Can you work these out from the model? Positions are in its coordinate system, mm. A direction names the side the tool comes from. Coordinates: 2 decimals unless noted, no trailing zeros. Order: outer loops, then holes, each group sorted by start corner. A loop starts at its lowest first (then second) coordinate and runs counter-clockwise, first axis right, second up. Notation, with made-up numbers: (42.25, 7.25) - (98.25, 7.25) arc R24 cw to (98.25, 34.25) - close; hole circle Ø8 at (15, 18.5). An arc over 180 degrees is marked (long way). Return JSON: item names as keys, results as strings. Group by question number.
1) Imagine slicing it at A-A (x = -30.48). Write out the boundary of the cut face in (y, z), and give its area (3 significant figures).
2) If I drill on line 1 along Z through (x, y) = (-30.5, 2); line 2 along Z through (x, y) = (-55, 20); line 3 along X through (y, z) = (12.5, 24), over which ranges is the centre line in solid material (lowest first)?
3) Imagine slicing it at D-D (y = 24). Write out the boundary of the cut face in (x, z), and give its area (3 significant figures).
4) Which directions (+Z, -Z, +X, -X, +Y, -Y) give clear straight access to the entire face, cutting with the end or side of a thin tool? Please do faces 1 (the face through (-38.1, 3, -12)), 2 (the face through (-41, 12.7, 13)), 3 (the face through (-60.07, 21.38, 13.27)).
5) For pin 1 Ø4 at (x, z) = (-30.5, -22) entering from -Y; pin 2 Ø1 at (y, z) = (9, -31) entering from +X; pin 3 Ø12.5 at (x, y) = (-56.5, 11.5) entering from +Z; pin 4 Ø6.5 at (x, z) = (-30.48, 25.4) entering from +Y, each with a flat end and sliding along its axis, tell me the tip position at first contact or that it passes through.
6) Imagine slicing it at B-B (y = 14.5). Write out the boundary of the cut face in (x, z), and give its area (3 significant figures).
7) Imagine slicing it at C-C (x = -49.5). Write out the boundary of the cut face in (y, z), and give its area (3 significant figures).
8) If we mould it in two halves opening along Z, with no side actions, what happens to faces 4 (the face through (-38.1, 3, 38)), 5 (the face through (-19, 3, 50.8)), 6 (the face through (-8.992, 1.805, -27.552))? For each: pulls with the +Z half, pulls with the -Z half, needs draft (parallel to the pull), parting line crosses it, or undercut.
```python
from build123d import *

# Parameters (mm, degrees)
EXTRUDE_THIN1_DEPTH                             = 50.8
CUT_EXTRUDE2_START                              = -7.35
SKETCH3_W                                       = 25.4
SKETCH3_H                                       = 25.4
CUT_EXTRUDE2_DEPTH                              = 27.4
LPATTERN1_COUNT                                 = 2
LPATTERN1_PITCH                                 = 50
CSK_FOR_10_FLAT_HEAD_MACHINE_SCREW1_D           = 5.1054
CSK_FOR_10_FLAT_HEAD_MACHINE_SCREW1_CSINK_D     = 9.779
CSK_FOR_10_FLAT_HEAD_MACHINE_SCREW1_CSINK_ANGLE = 82
LPATTERN2_COUNT                                 = 2
LPATTERN2_PITCH                                 = 50.8
LPATTERN2_COUNT_DIR2                            = 2
LPATTERN2_PITCH_DIR2                            = 22.86


with BuildPart() as part:
    # Sketch1 → Extrude-Thin1 (new body, symmetric)
    with BuildSketch(Plane.XY):
        with BuildLine():
            Line((0, 0), (-50.8, 0))
            ThreePointArc((-50.8, 0), (-59.780256121, 21.680256121), (-38.1, 12.7))
            Line((-38.1, 12.7), (-44.45, 12.7))
            ThreePointArc((-44.45, 12.7), (-55.290128061, 17.190128061), (-50.8, 6.35))
            Line((-50.8, 6.35), (0, 6.35))
            Line((0, 6.35), (0, 0))
        make_face()
    extrude(amount=EXTRUDE_THIN1_DEPTH, both=True)

    # Sketch3 → Cut-Extrude2 (cut)
    with BuildSketch(Plane(origin=(0, 6.35, 0), x_dir=(1, 0, 0), z_dir=(0, 1, 0)).offset(CUT_EXTRUDE2_START)):
        with Locations((-50.8, -38.1)):
            Rectangle(SKETCH3_W, SKETCH3_H)
    cut_extrude2 = extrude(amount=CUT_EXTRUDE2_DEPTH, mode=Mode.SUBTRACT)

    # LPattern1: Cut-Extrude2 ×2
    with Locations(*[(0, 0, -i * LPATTERN1_PITCH) for i in range(1, LPATTERN1_COUNT)]):
        add(cut_extrude2, mode=Mode.SUBTRACT)

    # CSK for #10 Flat Head Machine Screw1 (through all)
    with Locations(Plane(origin=(0, 6.35, 0), x_dir=(1, 0, 0), z_dir=(0, 1, 0))):
        with Locations((-30.48, 25.4)):
            csk_for_10_flat_head_machine_screw1 = CounterSinkHole(CSK_FOR_10_FLAT_HEAD_MACHINE_SCREW1_D / 2, CSK_FOR_10_FLAT_HEAD_MACHINE_SCREW1_CSINK_D / 2, counter_sink_angle=CSK_FOR_10_FLAT_HEAD_MACHINE_SCREW1_CSINK_ANGLE)

    # LPattern2: CSK for _10 Flat Head Machine Screw1 2 × 2
    with Locations(*[(j * LPATTERN2_PITCH_DIR2, 0, i * LPATTERN2_PITCH) for i in range(LPATTERN2_COUNT) for j in range(LPATTERN2_COUNT_DIR2) if (i, j) != (0, 0)]):
        add(csk_for_10_flat_head_machine_screw1, mode=Mode.SUBTRACT)


solid = part.part
```
Calculated:
{
 "1": {"outline": "(0, -50.8) - (6.35, -50.8) - (6.35, -30.29) - (3.66, -27.95) - (0, -27.95) - close; (0, -22.85) - (3.66, -22.85) - (6.35, -20.51) - (6.35, 20.51) - (3.66, 22.85) - (0, 22.85) - close; (0, 27.95) - (3.66, 27.95) - (6.35, 30.29) - (6.35, 50.8) - (0, 50.8) - close", "area": "568 mm2"},
 "2": {"line 1": "-50.8 to -27.95, -22.85 to 22.85, 27.95 to 50.8", "line 2": "-50.8 to -24.6, 0.8 to 25.4", "line 3": "-63.5 to -57.15"},
 "3": {"outline": "(-56.6, -50.8) - (-45, -50.8) - (-45, -24.6) - (-56.6, -24.6) - close; (-56.6, 0.8) - (-45, 0.8) - (-45, 25.4) - (-56.6, 25.4) - close", "area": "589 mm2"},
 "4": {"face 1": "-X, +Y, -Y", "face 2": "+Z, -Z, +X", "face 3": "+Z, -Z"},
 "5": {"pin 1": "y = 0", "pin 2": "x = -55.56", "pin 3": "z = 25.4", "pin 4": "y = 4.46"},
 "6": {"outline": "(-63.37, -50.8) - (-56.89, -50.8) - (-56.89, -24.6) - (-63.37, -24.6) - close; (-63.37, 0.8) - (-56.89, 0.8) - (-56.89, 25.4) - (-63.37, 25.4) - close; (-44.71, -50.8) - (-38.23, -50.8) - (-38.23, -24.6) - (-44.71, -24.6) - close; (-44.71, 0.8) - (-38.23, 0.8) - (-38.23, 25.4) - (-44.71, 25.4) - close", "area": "659 mm2"},
 "7": {"outline": "(0, -50.8) - (6.35, -50.8) - (6.35, -24.6) - (0, -24.6) - close; (0, 0.8) - (6.35, 0.8) - (6.35, 25.4) - (0, 25.4) - close; (18.92, -50.8) - (25.33, -50.8) - (25.33, -24.6) - (18.92, -24.6) - close; (18.92, 0.8) - (25.33, 0.8) - (25.33, 25.4) - (18.92, 25.4) - close", "area": "649 mm2"},
 "8": {"face 4": "needs draft", "face 5": "pulls with the +Z half", "face 6": "undercut"}
}
